from build123d import *

# Parameters (mm, degrees)
F0_W     = 431.8
F0_H     = 279.4
F1_DEPTH = 762
F2_W     = 76.2
F2_H     = 279.4
F3_DEPTH = 609.6
F5_DEPTH = 431.801


with BuildPart() as f1:
    # F0 (on Front) → F1 (new body)
    with BuildSketch(Plane.XZ):
        Rectangle(F0_W, F0_H)
    extrude(amount=F1_DEPTH)

    # F2 (on face) → F3 (cut)
    with BuildSketch(Plane(origin=(0, 0, 0), x_dir=(-1, 0, 0), z_dir=(0, 1, 0))):
        with Locations((-177.8, 0)):
            Rectangle(F2_W, F2_H)
    extrude(amount=-F3_DEPTH, mode=Mode.SUBTRACT)

    # F4 (on face) → F5 (cut, through all)
    with BuildSketch(Plane.YZ.offset(215.9)):
        Polygon((-762, 139.7), (-762, 84.815077), (-609.6, 84.815077), (-457.2, 140.538976), align=None)
        Polygon((-762, -84.815077), (-762, -139.7), (-457.2, -140.538976), (-609.6, -84.815077), align=None)
    extrude(amount=-F5_DEPTH, mode=Mode.SUBTRACT)


solid = f1.part
The model under review builds one solid part; all positions refer to its coordinate system, in mm. A direction names the side the tool comes from. Coordinates: 2 decimals unless noted, no trailing zeros. Write each loop counter-clockwise with the first axis right and the second up, starting at its lowest first coordinate (ties: lowest second). Pieces come first, ordered by that corner, then holes. Notation, with made-up numbers: M 26,71 L 79,71 A11 cw 79,86 Z; hole C 63.5,14 d7. An arc over 180 degrees is marked long. Put each result on its own line as item: value.
1) Wall thickness on probe 1 along X at (y, z) = (-522.5, 60); probe 2 along Z at (x, y) = (163.5, -620.5); probe 3 along Y at (x, z) = (165, 84): over which ranges is each line inside the solid? List them lowest first. Write a range as [from, to].
Computed:
probe 1: x = [-215.9, 139.7]
probe 2: z = [-84.82, 84.82]
probe 3: y = [-762, -609.6]
2) Add section A-A on z = -26.5. Give the boundary of the cut face in (x, y), then the cut area to 3 significant figures.
Computed:
outline: M -215.9,-762 L 215.9,-762 L 215.9,-609.6 L 139.7,-609.6 L 139.7,0 L -215.9,0 Z
area: 283,000 mm2
3) Clearance check with a flat-ended pin moving along its axis: pin 1 Ø10 at (y, z) = (-558.5, 53) entering from +X. State where the tip first meets the part, or that it passes through.
Computed:
pin 1: stops at x = 139.7
4) Add section D-D on x = 154. Give the boundary of the cut face in (y, z).
Computed:
outline: M -762,-84.82 L -609.6,-84.82 L -609.6,84.82 L -762,84.82 Z
5) For faces 1 (the flat face through (178, -609.6, 1)), 2 (the flat face through (3, -687, 84.815)), 3 (the flat face through (3, -685, -84.815)), list the 3-axis set-ups (+Z, -Z, +X, -X, +Y, -Y) from which the entire face can be reached by the end or side of a thin tool; tool diameter is ignored.
Computed:
face 1: +Z, -Z, +X, +Y
face 2: +Z, +X, -X, -Y
face 3: -Z, +X, -X, -Y
6) Add section B-B on x = -74. Give the boundary of the cut face in (y, z), then the cut area to 3 significant figures.
Computed:
outline: M -762,-84.82 L -609.6,-84.82 L -459.49,-139.7 L 0,-139.7 L 0,139.7 L -459.49,139.7 L -609.6,84.82 L -762,84.82 Z
area: 188,000 mm2
7) Add section C-C on y = -413. Give the boundary of the cut face in (x, z).
Computed:
outline: M -215.9,-139.7 L 139.7,-139.7 L 139.7,139.7 L -215.9,139.7 Z
